Here's how the part is built. I have some questions about the finished solid (model axes, mm). Coordinates: 2 decimals unless noted, no trailing zeros. Loops run counter-clockwise (first coordinate to the right, second up) from the corner with the lowest first, then second, coordinate; pieces in that order, holes last. Notation, with made-up numbers: (84.25, -6.75) -> (108.25, -6.75) arc R18 ccw to (108.25, 24.25) -> close; hole circle Ø6 at (-8.75, -29). An arc over 180 degrees is marked (long way). Answer as a JSON object with one key per item and string values. Group by question number.
Q1. I need wall thicknesses on line 1 (Y direction, x = 0, z = 5.75); line 2 (X direction, y = 2.5, z = 1.75); line 3 (Y direction, x = 3, z = 17). Which ranges of each line are inside material? Lowest first, please.
Q2. I'm going to push flat-ended pins straight in: pin 1 (8 mm diameter, centred on x = 13.5, z = 14.5, fed in from -Y); pin 2 (5 mm diameter, centred on y = -7.5, z = 15, fed in from -X); pin 3 (1.5 mm diameter, centred on y = 3, z = 3, fed in from +X). Where does each tip first touch, or does it pass through?
Q3. I want a section at B-B on z = 6. Write out the boundary of the cut face in (x, y).
Q4. Thinking about a two-plate mould opening in X: for faces 1 (the flat face through (13.05, 7.4, 8.9)), 2 (the flat face through (-12.93, 7.605, 8.897)), 3 (the cylindrical face through (6.944, -5.324, 8.874)), which applies, released by +X, released by -X, zero draft, split by the parting line, or undercut?
Q5. I want a section at A-A on x = 0. Write out the boundary of the cut face in (y, z).
```python
from build123d import *

# Parameters (mm, degrees)
EXTRUDE_1_DEPTH         = 18
HOLE_WIZARD_M20_1_D     = 17.5
HOLE_WIZARD_M20_1_DEPTH = 47.5
HOLE_WIZARD_M20_1_TIP   = 5.257530416


with BuildPart() as part:
    # 草图1 → 拉伸1 (new body)
    with BuildSketch(Plane.XY):
        Polygon((17.320508076, 0), (8.660254038, 15), (-8.660254038, 15), (-17.320508076, 0), (-8.660254038, -15), (8.660254038, -15), align=None)
    extrude(amount=EXTRUDE_1_DEPTH)

    # 草图2 → 切除-旋转1 (revolve, cut)
    with BuildSketch(Plane(origin=(0, 0, 0), x_dir=(1, 0, 0), z_dir=(0, 1, 0)), mode=Mode.PRIVATE) as cut_revolve_1_sk:
        Polygon((1.900444705, 5.902777738), (17.320508076, -3), (20.281011983, 2.127743183), align=None)
        Polygon((17.320508076, -15), (20.281011983, -20.127743183), (1.900444705, -23.902777738), align=None)
    revolve(cut_revolve_1_sk.sketch.rotate(Axis((0, 0, -13.306273389), (0, 0, 1)), 180), axis=Axis((0, 0, -13.306273389), (0, 0, 1)), mode=Mode.SUBTRACT)

    # M20 螺纹孔1
    with Locations(Plane.XY.offset(18)):
        with Locations((0, 0)):
            Hole(HOLE_WIZARD_M20_1_D / 2, depth=HOLE_WIZARD_M20_1_DEPTH)
            with Locations((0, 0, -(HOLE_WIZARD_M20_1_DEPTH + HOLE_WIZARD_M20_1_TIP / 2))):  # 118° drill point
                Cone(0, HOLE_WIZARD_M20_1_D / 2, HOLE_WIZARD_M20_1_TIP, mode=Mode.SUBTRACT)


solid = part.part
```
Result set:
{
 "1": {"line 1": "y = -15 to -8.75, 8.75 to 15", "line 2": "x = -14.95 to -8.39, 8.39 to 14.95", "line 3": "y = -13.53 to -8.22, 8.22 to 13.53"},
 "2": {"pin 1": "stops at y = -13.55", "pin 2": "stops at x = -14.43", "pin 3": "stops at x = 16.02"},
 "3": {"outline": "(-17.32, 0) -> (-8.66, -15) -> (8.66, -15) -> (17.32, 0) -> (8.66, 15) -> (-8.66, 15) -> close; hole circle Ø17.5 at (0, 0)"},
 "4": {"face 1": "released by +X", "face 2": "released by -X", "face 3": "undercut"},
 "5": {"outline": "(-15, 1.66) -> (-12.12, 0) -> (-8.75, 0) -> (-8.75, 18) -> (-12.12, 18) -> (-15, 16.34) -> close; (8.75, 0) -> (12.12, 0) -> (15, 1.66) -> (15, 16.34) -> (12.12, 18) -> (8.75, 18) -> close"}
}
